Autodesk Fusion 360 part; units mm, degrees
sketch "Skizze1" plane through (0, 0, 0) normal (0, 1, 0) x (1, 0, 0)
  line L0 (0, 0) -> (150, 0)
  line L1 (150, 0) -> (150, 70)
  line L2 (150, 70) -> (0, 70)
  line L3 (0, 70) -> (0, 0)
  dimension "d1" = 150
  dimension "d2" = 70
extrude "Extrusion1" add sketch "Skizze1" along normal blind 1.5
sketch "Skizze2" plane through (0, 1.5, 0) normal (0, 1, 0) x (-1, 0, 0)
  line L0 (0, -70) -> (0, 0)
  line L1 (0, 0) -> (-150, 0)
  line L2 (-150, 0) -> (-150, -70)
  line L3 (-150, -70) -> (0, -70)
  line L4 (-77, -55) -> (-130, -55) construction
  line L5 (-130, -55) -> (-130, -15) construction
  line L6 (-130, -15) -> (-77, -15) construction
  line L7 (-77, -15) -> (-77, -55) construction
  line L8 (-81.1558, -15) -> (-81.1558, -45) construction
  circle A0 centre (-130, -55) radius 2
  circle A1 centre (-77, -45) radius 2
  circle A2 centre (-77, -15) radius 2
  circle A3 centre (-130, -15) radius 2
  circle A4 centre (-25, -20) radius 6
  dimension "d5" = 53
  dimension "d6" = 40
  dimension "d7" = 20
  dimension "d8" = 15
  dimension "d10" = 4
  dimension "d11" = 4
  dimension "d12" = 4
  dimension "d13" = 4
  dimension "d14" = 12
  dimension "d17" = 30
extrude "Extrusion2" cut sketch "Skizze2" against normal blind 5 contours A0 | A1 | A2 | A3 | A4
Model file for the job. Use its own axes, mm. Give positions to 0.01 mm unless a question says otherwise; leave off trailing zeros. Order: outer loops, then holes, each group sorted by start corner. A loop starts at its lowest first (then second) coordinate and runs counter-clockwise, first axis right, second up.
1) Mould opens along Z. For faces 1 (the cylindrical face through (132, 1, -55)), 2 (the flat face through (74, 0, -35)) say: +Z half, -Z half, draft (parallel to the pull), parting line (faces both ways), or undercut.
2) Saw through at B-B, the plane z = -55. Write the cut outline in (x, y).
3) Pin check, flat tip, straight feed: pin 1 (2.5 mm diameter, centred on x = 130, z = -55, fed in from +Y). Stop position of the tip, or through.
4) Saw through at C-C, the plane x = 130. Write the cut outline in (y, z), then the cut area to 3 significant figures.
5) Wall check: probe 1 along Z at (x, y) = (77, 0.45); probe 2 along Z at (x, y) = (130, 1.2); probe 3 along Z at (x, y) = (25, 0.35). Give the ranges that are in metal, low to high.
6) Saw through at A-A, the plane x = 25. Write the cut outline in (y, z), then the cut area to 3 significant figures.
7) Saw through at D-D, the plane y = 0.7. Write the cut outline in (x, z).
Computed:
1. face 1: undercut
1. face 2: draft
2. outline: (0, 0) - (128, 0) - (128, 1.5) - (0, 1.5) - close; (132, 0) - (150, 0) - (150, 1.5) - (132, 1.5) - close
3. pin 1: passes through
4. outline: (0, -70) - (1.5, -70) - (1.5, -57) - (0, -57) - close; (0, -53) - (1.5, -53) - (1.5, -17) - (0, -17) - close; (0, -13) - (1.5, -13) - (1.5, 0) - (0, 0) - close
4. area: 93.0 mm2
5. probe 1: z = -70 to -47, -43 to -17, -13 to 0
5. probe 2: z = -70 to -57, -53 to -17, -13 to 0
5. probe 3: z = -70 to -26, -14 to 0
6. outline: (0, -70) - (1.5, -70) - (1.5, -26) - (0, -26) - close; (0, -14) - (1.5, -14) - (1.5, 0) - (0, 0) - close
6. area: 87.0 mm2
7. outline: (0, -70) - (150, -70) - (150, 0) - (0, 0) - close; hole circle Ø12 at (25, -20); hole circle Ø4 at (77, -45); hole circle Ø4 at (77, -15); hole circle Ø4 at (130, -55); hole circle Ø4 at (130, -15)
